Autodesk Inventor part; units mm, degrees
ref_plane "YZ Plane" through (0, 0, 0) normal (1, 0, 0) x (0, 1, 0)
ref_plane "XZ Plane" through (0, 0, 0) normal (0, 1, 0) x (-1, 0, 0)
ref_plane "XY Plane" through (0, 0, 0) normal (0, 0, 1) x (1, 0, 0)
ref_plane "작업 평면1" through (0, 0, 0) normal (0, 0, 1) x (1, 0, 0)
sketch "스케치1" plane through (0, 0, 0) normal (0, 0, 1) x (1, 0, 0)
  circle A0 centre (-7.7782, -7.7782) radius 1.55
  circle A1 centre (7.7782, -7.7782) radius 1.55
  circle A2 centre (7.7782, 7.7782) radius 1.55
  circle A3 centre (-7.7782, 7.7782) radius 1.55
  circle A4 centre (0, 0) radius 5
  circle A5 centre (0, 0) radius 13.9
  circle A6 centre (0, 11) radius 1.55
  circle A7 centre (11, 0) radius 1.55
  circle A8 centre (0, -11) radius 1.55
  circle A9 centre (-11, 0) radius 1.55
  circle A10 centre (0, 0) radius 5.2
  circle A11 centre (0, 0) radius 13.9
  circle A12 centre (11, 0) radius 1.35
  circle A13 centre (7.7782, 7.7782) radius 1.35
  circle A14 centre (0, 11) radius 1.35
  circle A15 centre (-7.7782, 7.7782) radius 1.35
  circle A16 centre (-11, 0) radius 1.35
  circle A17 centre (-7.7782, -7.7782) radius 1.35
  circle A18 centre (0, -11) radius 1.35
  circle A19 centre (7.7782, -7.7782) radius 1.35
  dimension "d0" = 0.2
  dimension "d1" = 2.7
  dimension "d4" = 360
extrude "돌출1" add sketch "스케치1" along normal blind 6 contours A5
properties part number "64horn" material "PMMA 플라스틱"
The model under review builds one solid part; all positions refer to its coordinate system, in mm. Coordinates: 2 decimals unless noted, no trailing zeros. Write each loop counter-clockwise with the first axis right and the second up, starting at its lowest first coordinate (ties: lowest second). Pieces come first, ordered by that corner, then holes. Notation, with made-up numbers: (-34, -18.75) - (-7, -18.75) arc R27 cw to (-7, 17.25) - close; hole circle Ø3 at (48, -28.5). An arc over 180 degrees is marked (long way). Answer in a Markdown table with one row per item. Add a question column.
Q1. Draft analysis for pull direction X (two halves, no side actions). For faces 1 (the face through (-3.01, 13.57, 2.96)), 2 (the face through (-0.677, -5.156, 2.958)), 3 (the face through (0, -6, 0)), state which applies: +X half, -X half, draft (parallel to the pull), parting line (faces both ways), or undercut.
Q2. Consider section D-D on y = -12. Give the boundary of the cut face in (x, z), then the cut area to 3 significant figures.
Q3. To check wall thickness, follow line 1 along Y through (x, z) = (0, 3.65); line 2 along X through (y, z) = (-0.5, 1.65); line 3 along Y through (x, z) = (9, 5.25). State the ranges of each line that lie inside material, in increasing order. Write a range as from..to.
Q4. Consider section A-A on x = 0. Give the boundary of the cut face in (y, z).
Q5. Consider section C-C on x = 11. Give the boundary of the cut face in (y, z).
Q6. Clearance check with a flat-ended pin moving along its axis: pin 1 (3 mm diameter, centred on x = -7.78, y = -7.78, fed in from -Z). State where the tip first meets the part, or that it passes through.
Answers below:
| question | item | result |
|---|---|---|
| 1 | face 1 | parting line |
| 1 | face 2 | undercut |
| 1 | face 3 | draft |
| 2 | outline | (-7.01, 0) - (-1.18, 0) - (-1.18, 6) - (-7.01, 6) - close; (1.18, 0) - (7.01, 0) - (7.01, 6) - (1.18, 6) - close |
| 2 | area | 70.0 mm² |
| 3 | line 1 | -13.9..-12.55, -9.45..-5.2, 5.2..9.45, 12.55..13.9 |
| 3 | line 2 | -13.89..-12.47, -9.53..-5.18, 5.18..9.53, 12.47..13.89 |
| 3 | line 3 | -10.59..-8.73, -6.82..6.82, 8.73..10.59 |
| 4 | outline | (-13.9, 0) - (-12.55, 0) - (-12.55, 6) - (-13.9, 6) - close; (-9.45, 0) - (-5.2, 0) - (-5.2, 6) - (-9.45, 6) - close; (5.2, 0) - (9.45, 0) - (9.45, 6) - (5.2, 6) - close; (12.55, 0) - (13.9, 0) - (13.9, 6) - (12.55, 6) - close |
| 5 | outline | (-8.5, 0) - (-1.55, 0) - (-1.55, 6) - (-8.5, 6) - close; (1.55, 0) - (8.5, 0) - (8.5, 6) - (1.55, 6) - close |
| 6 | pin 1 | through |
